Model file for the job. Use its own axes, mm. Face numbers are marked on the shaded views. A direction names the side the tool comes from. Coordinates: 2 decimals unless noted, no trailing zeros. Write each loop counter-clockwise with the first axis right and the second up, starting at its lowest first coordinate (ties: lowest second). Pieces come first, ordered by that corner, then holes. Notation, with made-up numbers: (58, -33.75) -> (108, -33.75) arc R21 ccw to (108, 3.25) -> close; hole circle Ø11 at (-13.75, 56.25). An arc over 180 degrees is marked (long way). Write item = value, one per line. Start each with the question number.
from build123d import *

# Parameters (mm, degrees)
SKETCH1_W                      = 296
SKETCH1_H                      = 200
BASE_FLANGE1_DEPTH             = 8
EDGE_FLANGE1_STRIP_W           = 52
EDGE_FLANGE1_STRIP_H           = 8
EDGE_FLANGE1_STRIP_CUT_DEPTH   = 200
EDGE_FLANGE1_STRIP_2_W         = 52
EDGE_FLANGE1_STRIP_2_H         = 8
EDGE_FLANGE1_STRIP_CUT_2_DEPTH = 200
EDGE_FLANGE1_DEPTH             = 200
EDGE_FLANGE1_BEND_DEPTH        = 200
SKETCH12_R                     = 30
CUT_EXTRUDE1_DEPTH             = 10
SKETCH13_R                     = 7.5
CUT_EXTRUDE2_DEPTH             = 10
SKETCH15_R                     = 7.5
CUT_EXTRUDE3_DEPTH             = 317.733326317
SKETCH16_R                     = 4.5
CUT_EXTRUDE4_DEPTH             = 10
MIRROR5_COPY_1_SKETCH_R        = 7.5
MIRROR5_COPY_1_DEPTH           = 10


# Sheet-metal steps are written as plain solids
with BuildPart() as part:
    # Sketch1 → Base-Flange1 (new body)
    with BuildSketch(Plane(origin=(0, 0, 0), x_dir=(1, 0, 0), z_dir=(0, 1, 0))):
        Rectangle(SKETCH1_W, SKETCH1_H)
    extrude(amount=-BASE_FLANGE1_DEPTH)

    # Edge-Flange1 strip (across the edge) → Edge-Flange1 strip cut (cut)
    with BuildSketch(Plane(origin=(-148, 0, -100), x_dir=(1, 0, 0), z_dir=(0, 0, 1))):
        with Locations((-8, -4)):
            Rectangle(EDGE_FLANGE1_STRIP_W, EDGE_FLANGE1_STRIP_H)
    extrude(amount=EDGE_FLANGE1_STRIP_CUT_DEPTH, mode=Mode.SUBTRACT)

    # Edge-Flange1 strip 2 (across the edge) → Edge-Flange1 strip cut 2 (cut)
    with BuildSketch(Plane(origin=(148, 0, 100), x_dir=(-1, 0, 0), z_dir=(0, 0, -1))):
        with Locations((-8, -4)):
            Rectangle(EDGE_FLANGE1_STRIP_2_W, EDGE_FLANGE1_STRIP_2_H)
    extrude(amount=EDGE_FLANGE1_STRIP_CUT_2_DEPTH, mode=Mode.SUBTRACT)

    # Edge-Flange1 section (across the edge) → Edge-Flange1 (add)
    with BuildSketch(Plane(origin=(-148, 0, -100), x_dir=(1, 0, 0), z_dir=(0, 0, 1))):
        with BuildLine():
            Line((0, 10), (0, 52))
            Line((0, 52), (8, 52))
            Line((8, 52), (8, 10))
            ThreePointArc((8, 10), (10.928932188, 2.928932188), (18, 0))
            Line((18, 0), (18, -8))
            ThreePointArc((18, -8), (5.272077939, -2.727922061), (0, 10))
        make_face()
    extrude(amount=EDGE_FLANGE1_DEPTH)

    # Edge-Flange1 section 2 (across the edge) → Edge-Flange1 bend (add)
    with BuildSketch(Plane(origin=(148, 0, 100), x_dir=(-1, 0, 0), z_dir=(0, 0, -1))):
        with BuildLine():
            Line((0, 10), (0, 52))
            Line((0, 52), (8, 52))
            Line((8, 52), (8, 10))
            ThreePointArc((8, 10), (10.928932188, 2.928932188), (18, 0))
            Line((18, 0), (18, -8))
            ThreePointArc((18, -8), (5.272077939, -2.727922061), (0, 10))
        make_face()
    extrude(amount=EDGE_FLANGE1_BEND_DEPTH)

    # Sketch12 → Cut-Extrude1 (cut)
    with BuildSketch(Plane(origin=(0, -8, 0), x_dir=(-1, 0, 0), z_dir=(0, -1, 0))):
        with Locations(Location((0, 0, 0), (0, 0, 90))):
            Circle(SKETCH12_R)
    extrude(amount=-CUT_EXTRUDE1_DEPTH, mode=Mode.SUBTRACT)

    # Sketch13 → Cut-Extrude2 (cut)
    with BuildSketch(Plane(origin=(0, -8, 0), x_dir=(-1, 0, 0), z_dir=(0, -1, 0))):
        with Locations(Location((55.437171645, -55.437171645, 0), (0, 0, 90))):
            Circle(SKETCH13_R)
    cut_extrude2 = extrude(amount=-CUT_EXTRUDE2_DEPTH, mode=Mode.SUBTRACT)

    # Mirror4: Cut-Extrude2 across plane
    add(cut_extrude2.mirror(Plane(origin=(0, 0, 0), x_dir=(0, 0, 1), z_dir=(1, 0, 0))), mode=Mode.SUBTRACT)

    # Sketch15 → Cut-Extrude3 (cut, through all)
    with BuildSketch(Plane.ZY.offset(148)):
        with Locations(Location((-60, 31, 0), (0, 0, 270))):
            Circle(SKETCH15_R)
    cut_extrude3 = extrude(amount=-CUT_EXTRUDE3_DEPTH, mode=Mode.SUBTRACT)

    # Sketch16 → Cut-Extrude4 (cut)
    with BuildSketch(Plane(origin=(0, -8, 0), x_dir=(-1, 0, 0), z_dir=(0, -1, 0))):
        with Locations(Location((105, 65, 0), (0, 0, 90))):
            Circle(SKETCH16_R)
    cut_extrude4 = extrude(amount=-CUT_EXTRUDE4_DEPTH, mode=Mode.SUBTRACT)

    # Mirror5: Cut-Extrude2, Cut-Extrude3, Cut-Extrude4 across plane
    add(cut_extrude2.mirror(Plane.XY), mode=Mode.SUBTRACT)
    add(cut_extrude3.mirror(Plane.XY), mode=Mode.SUBTRACT)
    add(cut_extrude4.mirror(Plane.XY), mode=Mode.SUBTRACT)

    # Mirror5 copy 1 sketch → Mirror5 copy 1 (cut)
    with BuildSketch(Plane.XZ.offset(8)):
        with Locations(Location((55.437171645, -55.437171645, 0), (0, 0, 90))):
            Circle(MIRROR5_COPY_1_SKETCH_R)
    extrude(amount=-MIRROR5_COPY_1_DEPTH, mode=Mode.SUBTRACT)


solid = part.part
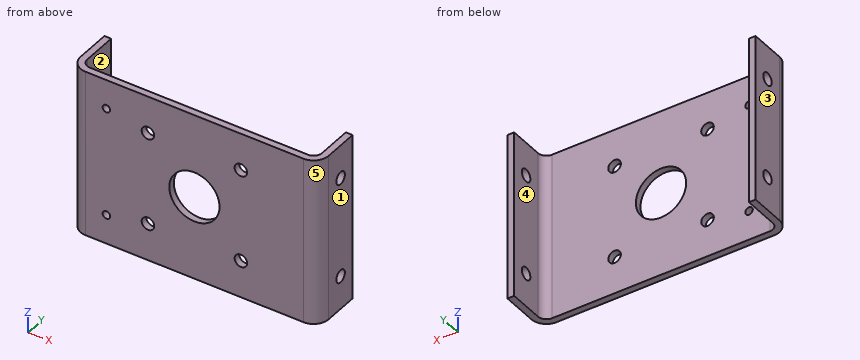
(1) Saw through at B-B (y = 45.5). Give the cut face in (x, z), then the cut area to 3 significant figures.
(2) Mould opens along X. For the marked faces 1, 2 and 3 say: released by +X, released by -X, zero draft, split by the parting line, or undercut.
(3) 3-axis set-ups, long thin cutter, end or side, ignore diameter. For the marked faces 4 and 5: which of +Z, -Z, +X, -X, +Y, -Y reach the whole face in a straight line?
(4) Drill centre lines: line 1 along Z through (x, y) = (145.5, 31); line 2 along X through (y, z) = (38, -69); line 3 along X through (y, z) = (9, -81.5). Where is each one in solid material? Low to high.
(5) Drop flat-ended pins along their axis: pin 1 Ø2 at (y, z) = (0.5, -20) entering from -X; pin 2 Ø17 at (x, z) = (-55.44, 55.44) entering from +Y; pin 3 Ø6 at (y, z) = (-1.5, 27) entering from +X. Give the stop position or say it passes through.
(6) Saw through at A-A (x = -105). Give the cut face in (y, z).
(7) Saw through at C-C (x = 0). Give the cut face in (y, z), then the cut area to 3 significant figures.
(8) Saw through at D-D (z = -35). Give the cut face in (x, y).
Returned:
q1.outline = (-148, -100) -> (-140, -100) -> (-140, 100) -> (-148, 100) -> close; (140, -100) -> (148, -100) -> (148, 100) -> (140, 100) -> close
q1.area = 3,200 mm2
q2.face_1 = released by +X
q2.face_2 = undercut
q2.face_3 = released by -X
q3.face_4 = +Z, -Z, +Y
q3.face_5 = +Z, -Z, +X, -Y
q4.line_1 = -100 to -67.5, -52.5 to 52.5, 67.5 to 100
q4.line_2 = -148 to -140, 140 to 148
q4.line_3 = -147.97 to -139.95, 139.95 to 147.97
q5.pin_1 = -145.87
q5.pin_2 = 0
q5.pin_3 = 145.87
q6.outline = (-8, -100) -> (0, -100) -> (0, -69.5) -> (-8, -69.5) -> close; (-8, -60.5) -> (0, -60.5) -> (0, 60.5) -> (-8, 60.5) -> close; (-8, 69.5) -> (0, 69.5) -> (0, 100) -> (-8, 100) -> close
q7.outline = (-8, -100) -> (0, -100) -> (0, -30) -> (-8, -30) -> close; (-8, 30) -> (0, 30) -> (0, 100) -> (-8, 100) -> close
q7.area = 1,120 mm2
q8.outline = (-148, 10) arc R18 ccw to (-130, -8) -> (130, -8) arc R18 ccw to (148, 10) -> (148, 52) -> (140, 52) -> (140, 10) arc R10 cw to (130, 0) -> (-130, 0) arc R10 cw to (-140, 10) -> (-140, 52) -> (-148, 52) -> close
